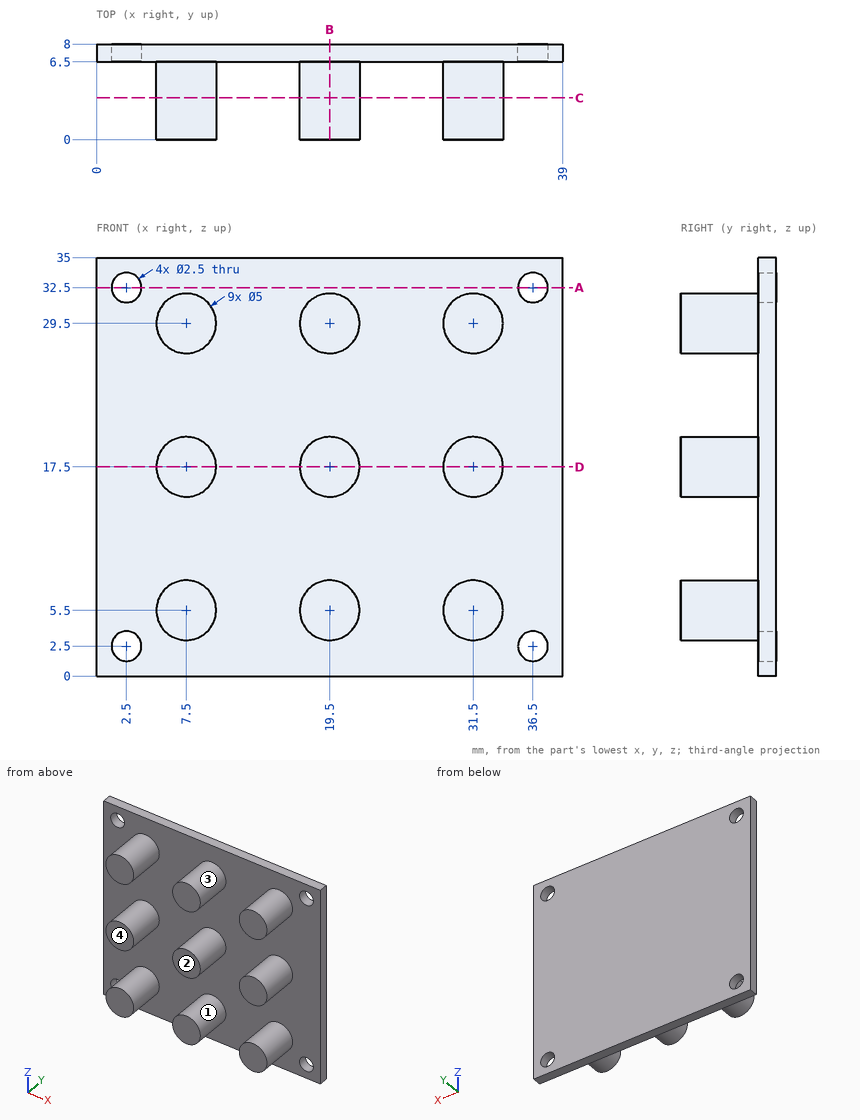
Could you check a few things on this drawing? It's one solid part, dimensions in mm from its lowest x, y, z. A direction names the side the tool comes from. Round coordinates to 2 decimals unless told otherwise and drop trailing zeros. Loops run counter-clockwise (first coordinate to the right, second up) from the corner with the lowest first, then second, coordinate; pieces in that order, holes last. Notation, with made-up numbers: (42, 65) -> (78, 65) arc R18 cw to (78, 79) -> close; hole circle Ø11 at (56, 48.5). An arc over 180 degrees is marked (long way). One line per item, written item: value. Start each with the question number.
1. If I drill on probe 1 along X at (y, z) = (6.85, 32.5); probe 2 along Z at (x, y) = (36.5, 7.15); probe 3 along Z at (x, y) = (7.5, 5), over which ranges is the centre line in solid material (lowest first)?
2. If we section it at A-A, the plane z = 32.5: Write out the boundary of the cut face in (x, y), then the cut area to 3 significant figures.
3. If we section it at B-B, the plane x = 19.5: Write out the boundary of the cut face in (y, z).
4. For pin 1 (3 mm diameter, centred on x = 2.5, z = 2.5, fed in from -Y); pin 2 (3 mm diameter, centred on x = 36.5, z = 32.5, fed in from +Y); pin 3 (1.5 mm diameter, centred on y = 5, z = 26, fed in from -X); pin 4 (4 mm diameter, centred on y = 3.5, z = 30.5, fed in from +X), each with a flat end and sliding along its axis, tell me the tip position at first contact or that it passes through.
5. For the marked faces 1 and 2, which set-ups out of +Z, -Z, +X, -X, +Y, -Y let a thin tool reach every point of the face, with its end or its side?
6. If we section it at C-C, the plane y = 3.5: Give the number of separate pieces and of enclosed holes in the cut face, then the cut area to 3 significant figures.
7. If we section it at D-D, the plane z = 17.5: Write out the boundary of the cut face in (x, y).
8. If we mould it in two halves opening along Z, with no side actions, what happens to the marked faces 3 and 4? For each: pulls with the +Z half, pulls with the -Z half, needs draft (parallel to the pull), parting line crosses it, or undercut.
Calculated:
1. probe 1: x = 0 to 1.25, 3.75 to 35.25, 37.75 to 39
1. probe 2: z = 0 to 1.25, 3.75 to 31.25, 33.75 to 35
1. probe 3: z = 3 to 8, 15 to 20, 27 to 32
2. outline: (0, 6.5) -> (1.25, 6.5) -> (1.25, 8) -> (0, 8) -> close; (3.75, 6.5) -> (35.25, 6.5) -> (35.25, 8) -> (3.75, 8) -> close; (37.75, 6.5) -> (39, 6.5) -> (39, 8) -> (37.75, 8) -> close
2. area: 51.0 mm²
3. outline: (0, 3) -> (6.5, 3) -> (6.5, 0) -> (8, 0) -> (8, 35) -> (6.5, 35) -> (6.5, 32) -> (0, 32) -> (0, 27) -> (6.5, 27) -> (6.5, 20) -> (0, 20) -> (0, 15) -> (6.5, 15) -> (6.5, 8) -> (0, 8) -> close
4. pin 1: stops at y = 6.5
4. pin 2: stops at y = 8
4. pin 3: passes through
4. pin 4: stops at x = 34
5. face 1: -Y
5. face 2: +Z, -Z, +X, -X, -Y
6. separate pieces: 9
6. enclosed holes: 0
6. area: 177 mm²
7. outline: (0, 6.5) -> (5, 6.5) -> (5, 0) -> (10, 0) -> (10, 6.5) -> (17, 6.5) -> (17, 0) -> (22, 0) -> (22, 6.5) -> (29, 6.5) -> (29, 0) -> (34, 0) -> (34, 6.5) -> (39, 6.5) -> (39, 8) -> (0, 8) -> close
8. face 3: undercut
8. face 4: needs draft
